Design review of the part shown in the three views and the two pictorial views. Dimensions are in mm from the part's minimum x, y and z. Round coordinates to 2 decimals unless told otherwise and drop trailing zeros. Loops run counter-clockwise (first coordinate to the right, second up) from the corner with the lowest first, then second, coordinate; pieces in that order, holes last. Notation, with made-up numbers: M 5.5,61.25 L 44.5,61.25 A22 cw 44.5,71.25 Z; hole C 89,66 d6. An arc over 180 degrees is marked long. One line per question, with ' | ' between items.
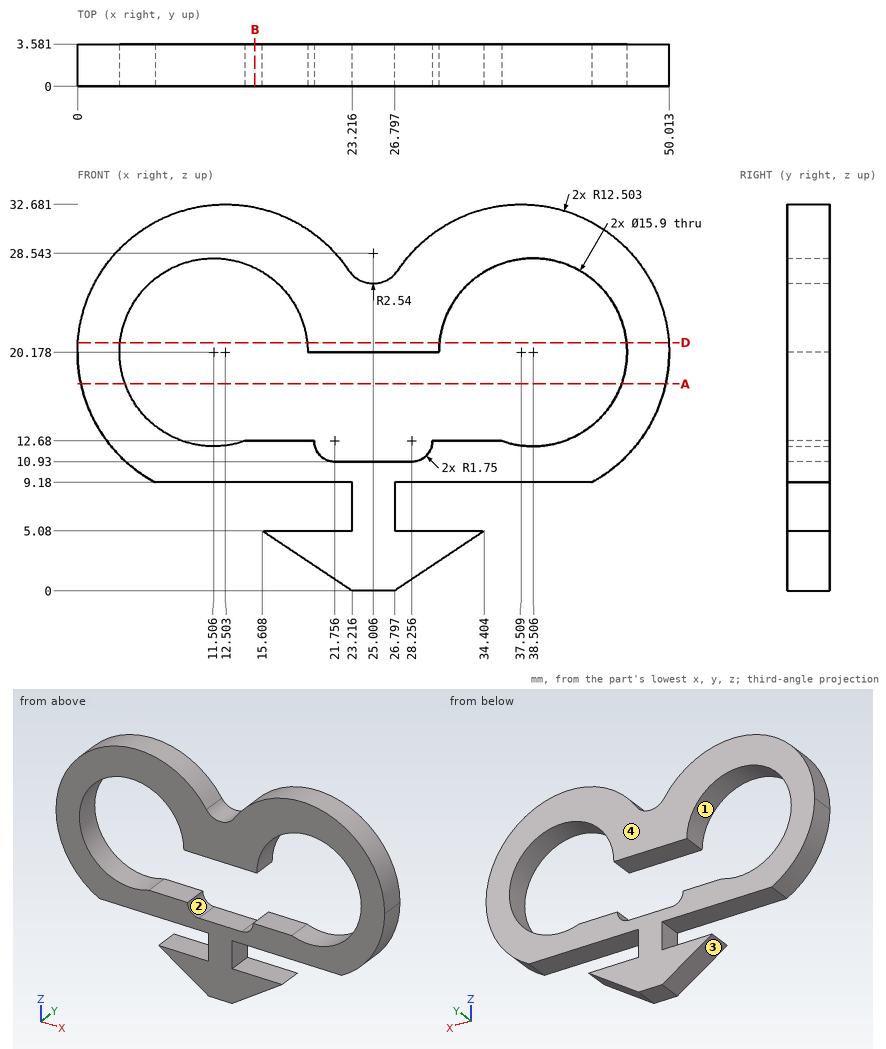
1) Add section B-B on x = 15. State the section outline as (y, z) points.
Output values:
outline: M 0,9.18 L 3.58,9.18 L 3.58,12.68 L 0,12.68 Z; M 0,27.32 L 3.58,27.32 L 3.58,32.43 L 0,32.43 Z
2) Insertion check: P1, Ø14.5, axis at x = 38.51, z = 20.18, coming from the -Y side; P2, Ø1.8, axis at x = 31, y = 2.5, coming from the +Z side; P3, Ø1.8, axis at x = 32.5, y = 2.5, coming from the -Z side; P4, Ø1.1, axis at x = 16, y = 1, coming from the +Z side. Each pin has a flat end and moves straight along its axis. Give the tip position at first contact, or say it passes through.
Output values:
P1: passes through | P2: stops at z = 31.35 | P3: stops at z = 3.21 | P4: stops at z = 32.33
3) For line 1 (Z direction, x = 33, y = 0.5) (1 decimal); line 2 (X direction, y = 1.9, z = 25) (1 decimal); line 3 (X direction, y = 1.85, z = 23) (1 decimal), list the stretches that pass through material, from the lowest coordinate up.
Output values:
line 1: z = 4.1 to 5.1, 9.2 to 12.7, 25.9 to 31.8 | line 2: x = 1 to 5.2, 17.8 to 32.2, 44.8 to 49 | line 3: x = 0.3 to 4.1, 18.9 to 31.1, 45.9 to 49.7
4) Add section D-D on z = 21. State the section outline as (x, y) points (1 decimal).
Output values:
outline: M 0,0 L 3.6,0 L 3.6,3.6 L 0,3.6 Z; M 19.4,0 L 30.6,0 L 30.6,3.6 L 19.4,3.6 Z; M 46.4,0 L 50,0 L 50,3.6 L 46.4,3.6 Z
5) Mouldability with a two-part tool opening along X and no side actions: class the marked faces 1, 2, 3 and 4 as +X half, -X half, draft (parallel to the pull), parting line (faces both ways), or undercut.
Output values:
face 1: undercut | face 2: undercut | face 3: -X half | face 4: draft
6) Add section A-A on z = 17.5. State the section outline as (x, y) points.
Output values:
outline: M 0.29,0 L 4.02,0 L 4.02,3.58 L 0.29,3.58 Z; M 45.99,0 L 49.72,0 L 49.72,3.58 L 45.99,3.58 Z
